```python
from build123d import *

# Parameters (mm, degrees)
F2_W     = 83.072104
F2_H     = 76.524554
F2_W_2   = 36.83
F2_H_2   = 36.83
F3_DEPTH = 81.534


with BuildPart() as f1:
    # F0 (on Top) → F1 (revolve)
    with BuildSketch(Plane.XY):
        with BuildLine():
            Line((-5.780561, 67.105159), (-5.780561, 53.927373))
            Line((-5.780561, 53.927373), (-23.645375, 53.927373))
            Line((-23.645375, 53.927373), (-23.645375, 19.336753))
            Line((-23.645375, 19.336753), (0, 0))
            Line((0, 0), (0, 67.846416))
            Line((0, 67.846416), (0, 72.587589))
            ThreePointArc((0, 72.587589), (-4.06846, 71.088622), (-5.780561, 67.105159))
        make_face()
    revolve(axis=Axis((0, 33.923208, 0), (0, -1, 0)))

    # F2 (on Front) → F3 (cut)
    with BuildSketch(Plane.XZ):
        Rectangle(F2_W, F2_H)
        Rectangle(F2_W_2, F2_H_2, mode=Mode.SUBTRACT)
    extrude(amount=-F3_DEPTH, mode=Mode.SUBTRACT)


solid = f1.part
```
Part model, mm, in its own coordinate system. A direction names the side the tool comes from. Round coordinates to 2 decimals unless told otherwise and drop trailing zeros. Loops run counter-clockwise (first coordinate to the right, second up) from the corner with the lowest first, then second, coordinate; pieces in that order, holes last.
Item 1: Cut at C-C, the plane y = 63. Give the cut face in (x, z).
Item 2: 3-axis set-ups, long thin cutter, end or side, ignore diameter. For faces 1 (the face through (-16.745, 36.39, -16.695)), 2 (the face through (-4.4, 53.927, -4.4)): which of +Z, -Z, +X, -X, +Y, -Y reach the whole face in a straight line?
Item 3: Drill centre lines: line 1 (Y direction, x = -10, z = 15); line 2 (X direction, y = 25, z = -15); line 3 (Z direction, x = -3.5, y = 57). Where is each one in solid material? Low to high.
Item 4: Drop flat-ended pins along their axis: P1, Ø1.5, axis at x = 13, z = -6.5, coming from the -Y side; P2, Ø3, axis at x = -6, z = 8, coming from the -Y side; P3, Ø4, axis at x = -3.5, z = 12, coming from the -Y side. Give the stop position or say it passes through.
Item 5: Cut at A-A, the plane y = 25.5. Give the cut face in (x, z) (3 decimals), then the cut area to 3 significant figures.
Item 6: Cut at B-B, the plane y = 12. Give the cut face in (x, z).
A:
1. outline: circle Ø11.56 at (0, 0)
2. face 1: -Z, -X, +Y, -Y
2. face 2: +Y
3. line 1: y = 14.74 to 53.93
3. line 2: x = -18.28 to 18.28
3. line 3: z = -4.6 to 4.6
4. P1: stops at y = 11.27
4. P2: stops at y = 6.95
4. P3: stops at y = 8.59
5. outline: (-18.415, -14.832) arc R23.645 ccw to (-14.832, -18.415) - (14.832, -18.415) arc R23.645 ccw to (18.415, -14.832) - (18.415, 14.832) arc R23.645 ccw to (14.832, 18.415) - (-14.832, 18.415) arc R23.645 ccw to (-18.415, 14.832) - close
5. area: 1,330 mm2
6. outline: circle Ø29.35 at (0, 0)
